Check sheet for the modelled part. Datum: model origin and axes. Units: mm. A direction names the side the tool comes from. Round coordinates to 2 decimals unless told otherwise and drop trailing zeros. Write each loop counter-clockwise with the first axis right and the second up, starting at its lowest first coordinate (ties: lowest second). Pieces come first, ordered by that corner, then holes.
from build123d import *

# Parameters (mm, degrees)
F0_W      = 100
F0_H      = 100
F1_DEPTH  = 10
F2_W      = 10
F2_H      = 10
F3_DEPTH  = 10
F4_W      = 10
F4_H      = 20
F5_DEPTH  = 10
F6_W      = 10
F6_H      = 20
F7_DEPTH  = 10
F8_W      = 10
F8_H      = 20
F9_DEPTH  = 10
F10_W     = 20
F10_H     = 10
F11_DEPTH = 10
F12_W     = 20
F12_H     = 10
F13_DEPTH = 10
F14_W     = 20
F14_H     = 10
F15_DEPTH = 10
F16_W     = 10
F16_H     = 10
F17_DEPTH = 10
F18_W     = 10
F18_H     = 20
F19_DEPTH = 10
F20_W     = 10
F20_H     = 20
F21_DEPTH = 10
F22_W     = 10
F22_H     = 20
F23_DEPTH = 10


with BuildPart() as f1:
    # F0 (on Front) → F1 (new body)
    with BuildSketch(Plane.XZ):
        with Locations((3.271748, -2.17455)):
            Rectangle(F0_W, F0_H)
    extrude(amount=F1_DEPTH)

    # F2 (on face) → F3 (cut)
    with BuildSketch(Plane.XZ.offset(10)):
        with Locations((-41.728252, 42.82545)):
            Rectangle(F2_W, F2_H)
    extrude(amount=-F3_DEPTH, mode=Mode.SUBTRACT)

    # F4 (on face) → F5 (cut)
    with BuildSketch(Plane.XZ.offset(10)):
        with Locations((-41.728252, 17.82545)):
            Rectangle(F4_W, F4_H)
    extrude(amount=-F5_DEPTH, mode=Mode.SUBTRACT)

    # F6 (on face) → F7 (cut)
    with BuildSketch(Plane.XZ.offset(10)):
        with Locations((-41.728252, -12.17455)):
            Rectangle(F6_W, F6_H)
    extrude(amount=-F7_DEPTH, mode=Mode.SUBTRACT)

    # F8 (on face) → F9 (cut)
    with BuildSketch(Plane.XZ.offset(10)):
        with Locations((-41.728252, -42.17455)):
            Rectangle(F8_W, F8_H)
    extrude(amount=-F9_DEPTH, mode=Mode.SUBTRACT)

    # F10 (on face) → F11 (cut)
    with BuildSketch(Plane.XZ.offset(10)):
        with Locations((-26.728252, -47.17455)):
            Rectangle(F10_W, F10_H)
    extrude(amount=-F11_DEPTH, mode=Mode.SUBTRACT)

    # F12 (on face) → F13 (cut)
    with BuildSketch(Plane.XZ.offset(10)):
        with Locations((3.271748, -47.17455)):
            Rectangle(F12_W, F12_H)
    extrude(amount=-F13_DEPTH, mode=Mode.SUBTRACT)

    # F14 (on face) → F15 (cut)
    with BuildSketch(Plane.XZ.offset(10)):
        with Locations((33.271748, -47.17455)):
            Rectangle(F14_W, F14_H)
    extrude(amount=-F15_DEPTH, mode=Mode.SUBTRACT)

    # F16 (on face) → F17 (cut)
    with BuildSketch(Plane.XZ.offset(10)):
        with Locations((48.271748, 42.82545)):
            Rectangle(F16_W, F16_H)
    extrude(amount=-F17_DEPTH, mode=Mode.SUBTRACT)

    # F18 (on face) → F19 (cut)
    with BuildSketch(Plane.XZ.offset(10)):
        with Locations((48.271748, 17.82545)):
            Rectangle(F18_W, F18_H)
    extrude(amount=-F19_DEPTH, mode=Mode.SUBTRACT)

    # F20 (on face) → F21 (cut)
    with BuildSketch(Plane.XZ.offset(10)):
        with Locations((48.271748, -12.17455)):
            Rectangle(F20_W, F20_H)
    extrude(amount=-F21_DEPTH, mode=Mode.SUBTRACT)

    # F22 (on face) → F23 (cut)
    with BuildSketch(Plane.XZ.offset(10)):
        with Locations((48.271748, -42.17455)):
            Rectangle(F22_W, F22_H)
    extrude(amount=-F23_DEPTH, mode=Mode.SUBTRACT)


solid = f1.part
1. Set-up check for faces 4 (the flat face through (43.272, -5, -12)), 5 (the flat face through (-42, -5, 7.825)), 6 (the flat face through (-6.728, -5, -47)): record each of +Z, -Z, +X, -X, +Y, -Y from which the full face is reachable in a straight line by a thin tool's end or side.
2. Sectioned sample at B-B, the plane x = 36. Enter the section's corners in (y, z).
3. Release check for a two-part mould opening along X. For faces 1 (the flat face through (-42, -5, 27.825)), 2 (the flat face through (13.272, -5, -47)), 3 (the flat face through (43.272, -5, 43)) record: released by +X, released by -X, zero draft, split by the parting line, or undercut.
4. Sectioned sample at A-A, the plane z = 17.5. Enter the section's corners in (x, y), plus the area to 3 significant figures.
5. Go/stop test with flat-tipped pins: pin 1 (3 mm diameter, centred on x = -40, y = -5.5, fed in from -Z); pin 2 (6 mm diameter, centred on x = -35.5, y = -2.5, fed in from -Z); pin 3 (5 mm diameter, centred on x = -41, y = -2.5, fed in from +Z). Record where each tip stops, or that it passes through.
6. Scan lines: line 1 along Z through (x, y) = (45, -4); line 2 along X through (y, z) = (-6.75, -39); line 3 along Z through (x, y) = (31, -3.75). Record each from-to range of solid material in increasing order.
Computed values:
1. face 4: +X, +Y, -Y
1. face 5: -X, +Y, -Y
1. face 6: -Z, +Y, -Y
2. outline: (-10, -42.17) - (0, -42.17) - (0, 47.83) - (-10, 47.83) - close
3. face 1: zero draft
3. face 2: undercut
3. face 3: released by +X
4. outline: (-36.73, -10) - (43.27, -10) - (43.27, 0) - (-36.73, 0) - close
4. area: 800 mm2
5. pin 1: stops at z = -32.17
5. pin 2: stops at z = -42.17
5. pin 3: stops at z = 37.83
6. line 1: z = -32.17 to -22.17, -2.17 to 7.83, 27.83 to 37.83
6. line 2: x = -36.73 to 43.27
6. line 3: z = -42.17 to 47.83
